Input: part model. Units: mm. Frame: model coordinates. Round coordinates to 2 decimals unless told otherwise and drop trailing zeros. Loops run counter-clockwise (first coordinate to the right, second up) from the corner with the lowest first, then second, coordinate; pieces in that order, holes last. Notation, with made-up numbers: M 7.25,-25 L 26.25,-25 A16 cw 26.25,-2 Z; hole C -6.75,86.25 d3. An arc over 180 degrees is marked long. Return JSON: item names as keys, results as strings. Group by question number.
1) Material intervals for line 1 (Y direction, x = 547, z = -1.25); line 2 (Y direction, x = 252, z = -1.75); line 3 (X direction, y = 4, z = -1), sorted ascending. Write a range as from..to.
2) Section A-A (z = 0). Output: boundary loops of the cut face in (x, y), plus the area to 3 significant figures.
3) Section B-B (x = 443). Output: boundary loops of the cut face in (y, z), plus the area to 3 significant figures.
4) Contact query for flat-ended pins moving along their axis: P1, Ø2, axis at y = 1828, z = -2.5, coming from the +X side; P2, Ø3, axis at x = 487, z = -3.5, coming from the -Y side; P3, Ø6.5, axis at y = -100.5, z = 0, coming from the +X side; P4, Ø4, axis at x = 206.5, z = 1.5, coming from the -Y side. Output: stop coordinate, or through.
5) Section C-C (y = 528.5). Output: boundary loops of the cut face in (x, z).
from build123d import *

# Parameters (mm, degrees)
SWEEP1_PROFILE_R = 6.35


with BuildPart() as part:
    # Sweep1: sweep along a path in Sketch1
    with BuildLine(Plane.XY) as sweep1_path:
        Line((675, 2050), (75, 2050))
        ThreePointArc((75, 2050), (21.966991411, 2028.033008589), (0, 1975))
        Line((0, 1975), (0, 0))
        Line((0, 0), (0, -25))
        ThreePointArc((0, -25), (21.966991411, -78.033008589), (75, -100))
        Line((75, -100), (600, -100))
    # Sweep1 profile (on start of the path) → Sweep1 (sweep)
    with BuildSketch(Plane(origin=(675, 2050, 0), x_dir=(0, 0, -1), z_dir=(-1, 0, 0))):
        Circle(SWEEP1_PROFILE_R)
    sweep(path=sweep1_path.line)


solid = part.part
Returned:
{
 "1": {"line 1": "y = -106.23..-93.77, 2043.77..2056.23", "line 2": "y = -106.1..-93.9, 2043.9..2056.1", "line 3": "x = -6.27..6.27"},
 "2": {"outline": "M -6.35,-25 A81.35 ccw 75,-106.35 L 600,-106.35 L 600,-93.65 L 75,-93.65 A68.65 cw 6.35,-25 L 6.35,1975 A68.65 cw 75,2043.65 L 675,2043.65 L 675,2056.35 L 75,2056.35 A81.35 ccw -6.35,1975 Z", "area": "42,700 mm^2"},
 "3": {"outline": "C -100,0 d12.7; C 2050,0 d12.7", "area": "253 mm^2"},
 "4": {"P1": "stops at x = 6.17", "P2": "stops at y = -106.03", "P3": "stops at x = 600", "P4": "stops at y = -106.35"},
 "5": {"outline": "C 0,0 d12.7"}
}
